Model file for the job. Use its own axes, mm. Face numbers are marked on the shaded views. A direction names the side the tool comes from. Give positions to 0.01 mm unless a question says otherwise; leave off trailing zeros. Write each loop counter-clockwise with the first axis right and the second up, starting at its lowest first coordinate (ties: lowest second). Pieces come first, ordered by that corner, then holes.
```python
from build123d import *

# Parameters (mm, degrees)
F2_R    = 1.524
F3_SIZE = 0.762
F4_SIZE = 1.524


with BuildPart() as f1:
    # F0 (on Front) → F1 (revolve)
    with BuildSketch(Plane.XZ):
        Polygon((-31.75, 0), (0, 0), (0, 26.9875), (-12.7, 26.9875), (-12.7, 30.1625), (-19.05, 30.1625), (-19.05, 5.55625), (-31.75, 5.55625), align=None)
    revolve(axis=Axis((-15.875, 0, 0), (-1, 0, 0)))

    # F2
    f2_edges = [f1.edges().sort_by_distance(p)[0] for p in [
        (-19.05, 0, -5.55625),
    ]]
    fillet(f2_edges, radius=F2_R)

    # F3
    f3_edges = [f1.edges().sort_by_distance(p)[0] for p in [
        (-31.75, 0, -5.55625),
    ]]
    chamfer(f3_edges, length=F3_SIZE)

    # F4
    f4_edges = [f1.edges().sort_by_distance(p)[0] for p in [
        (0, 0, -26.9875),
    ]]
    chamfer(f4_edges, length=F4_SIZE)


solid = f1.part
```
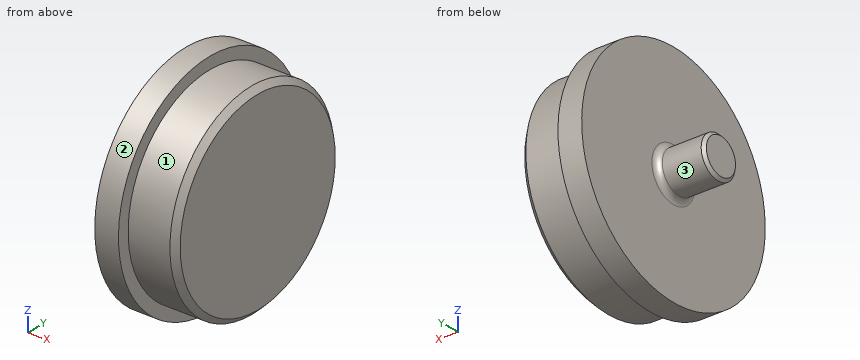
1. Probe probe 1 along X at (y, z) = (-5.5, 12.5); probe 2 along Z at (x, y) = (-29, -3.5); probe 3 along Z at (x, y) = (-8.5, 8.5). List the from-to ranges inside material, lowest first.
Calculated:
probe 1: x = -19.05 to 0
probe 2: z = -4.32 to 4.32
probe 3: z = -25.61 to 25.61
2. Which spindle directions (+Z, -Z, +X, -X, +Y, -Y) get a long thin tool onto all of the face, cutting with end or side? Do the marked faces 1, 2 and 3. Say none if no direction does.
Calculated:
face 1: +X
face 2: +X, -X
face 3: -X
3. Slice it at D-D, the plane x = -22. Write the cut outline in (y, z), and give its area (3 significant figures).
Calculated:
outline: circle Ø11.11 at (0, 0)
area: 97.0 mm2
4. Slice it at C-C, the plane x = -14. Write the cut outline in (y, z) (1 decimal), and give its area (3 significant figures).
Calculated:
outline: circle Ø60.3 at (0, 0)
area: 2,860 mm2
5. Pin check, flat tips, straight feed: P1, Ø12, axis at x = -6.5, y = -21.5, coming from the +Z side; P2, Ø4, axis at x = -17, z = -12, coming from the -Y side; P3, Ø1.5, axis at x = -10, y = 21.5, coming from the +Z side. Stop position of each tip, or through.
Calculated:
P1: stops at z = 22.09
P2: stops at y = -28.46
P3: stops at z = 17.26
6. Slice it at A-A, the plane y = 0. Write the cut outline in (x, z), and give its area (3 significant figures).
Calculated:
outline: (-31.75, -4.79) - (-30.99, -5.56) - (-20.57, -5.56) arc R1.52 cw to (-19.05, -7.08) - (-19.05, -30.16) - (-12.7, -30.16) - (-12.7, -26.99) - (-1.52, -26.99) - (0, -25.46) - (0, 25.46) - (-1.52, 26.99) - (-12.7, 26.99) - (-12.7, 30.16) - (-19.05, 30.16) - (-19.05, 7.08) arc R1.52 cw to (-20.57, 5.56) - (-30.99, 5.56) - (-31.75, 4.79) - close
area: 1,210 mm2
